```python
from build123d import *

# Parameters (mm, degrees)
F0_W           = 25.4
F0_H           = 76.2
F1_DEPTH       = 25.4
F2_W           = 25.4
F2_H           = 12.7
F3_DEPTH       = 6.35
F5_START       = -6.35
F4_R           = 9.525
F5_DEPTH       = 63.5
F6_R           = 5.1562
F7_DEPTH       = 76.201
F9_W           = 5.08
F9_H           = 76.2
F10_DEPTH      = 38.1
F11_W          = 20.32
F11_H          = 76.2
F12_DEPTH      = 6.35
F8_R           = 6.35
F13_DEPTH      = 5.6014842716
F13_DEPTH_BACK = 38.101


with BuildPart() as f1:
    # F0 (on Top) → F1 (new body)
    with BuildSketch(Plane.XY):
        with Locations((12.7, 38.1)):
            Rectangle(F0_W, F0_H)
    extrude(amount=F1_DEPTH)

    # F2 (on Top) → F3 (join)
    with BuildSketch(Plane.XY):
        with Locations((-12.7, 6.35)):
            Rectangle(F2_W, F2_H)
        with Locations((38.1, 6.35)):
            Rectangle(F2_W, F2_H)
        with Locations((-12.7, 69.85)):
            Rectangle(F2_W, F2_H)
        with Locations((38.1, 69.85)):
            Rectangle(F2_W, F2_H)
    extrude(amount=F3_DEPTH)

    # F4 (on face) → F5 (cut)
    with BuildSketch(Plane.XZ.offset(F5_START)):
        with Locations((12.7, 12.7)):
            Circle(F4_R)
    extrude(amount=-F5_DEPTH, mode=Mode.SUBTRACT)

    # F6 (on face) → F7 (cut, through all)
    with BuildSketch(Plane.XZ):
        with Locations((12.7, 12.7)):
            Circle(F6_R)
    extrude(amount=-F7_DEPTH, mode=Mode.SUBTRACT)

    # F9 (on face) → F10 (join)
    with BuildSketch(Plane.XY.offset(25.4)):
        with Locations((22.86, 38.1)):
            Rectangle(F9_W, F9_H)
        with Locations((2.54, 38.1)):
            Rectangle(F9_W, F9_H)
    extrude(amount=F10_DEPTH)

    # F11 (on face) → F12 (join)
    with BuildSketch(Plane.XY.offset(63.5)):
        with Locations((10.16, 38.1)):
            Rectangle(F11_W, F11_H)
    extrude(amount=-F12_DEPTH)

    # F8 (on face) → F13 (cut, two sides)
    with BuildSketch(Plane.XY.offset(25.4)) as f13_sk:
        with Locations((12.7, 38.1)):
            Circle(F8_R)
    extrude(amount=-F13_DEPTH, mode=Mode.SUBTRACT)
    extrude(f13_sk.sketch, amount=F13_DEPTH_BACK, mode=Mode.SUBTRACT)


solid = f1.part
```
Verification items for the finished model (mm, model axes). A direction names the side the tool comes from. Give positions to 0.01 mm unless a question says otherwise; leave off trailing zeros. Loops run counter-clockwise (first coordinate to the right, second up) from the corner with the lowest first, then second, coordinate; pieces in that order, holes last. Notation, with made-up numbers: M 19,56 L 36,56 A29 ccw 36,81 Z; hole C 34,88.25 d2. An arc over 180 degrees is marked long. One line per question, with ' | ' between items.
Item 1: Thickness scan on line 1 (X direction, y = 37.5, z = 30); line 2 (Z direction, x = 8.5, y = 59); line 3 (Z direction, x = 20, y = 46). Record the ranges inside material, lowest first. Write a range as [from, to].
Completed:
line 1: x = [0, 5.08], [20.32, 25.4] | line 2: z = [0, 4.15], [21.25, 25.4], [57.15, 63.5] | line 3: z = [0, 6.58], [18.82, 25.4], [57.15, 63.5]
Item 2: Section check B-B, the plane x = 33. Record the cut outline in (y, z).
Completed:
outline: M 0,0 L 12.7,0 L 12.7,6.35 L 0,6.35 Z; M 63.5,0 L 76.2,0 L 76.2,6.35 L 63.5,6.35 Z
Item 3: Section check A-A, the plane z = 12.7. Record the cut outline in (x, y) (3 decimals).
Completed:
outline: M 0,0 L 7.544,0 L 7.544,6.35 L 3.175,6.35 L 3.175,69.85 L 7.544,69.85 L 7.544,76.2 L 0,76.2 Z; M 17.856,0 L 25.4,0 L 25.4,76.2 L 17.856,76.2 L 17.856,69.85 L 22.225,69.85 L 22.225,6.35 L 17.856,6.35 Z
Item 4: Section check C-C, the plane y = 30. Record the cut outline in (x, z) (3 decimals).
Completed:
outline: M 0,0 L 25.4,0 L 25.4,63.5 L 0,63.5 Z; hole C 12.7,12.7 d19.05; hole M 5.08,25.4 L 20.32,25.4 L 20.32,57.15 L 5.08,57.15 Z
Item 5: Tool access check on faces 4 (the face through (19.4, 38.6, 57.15)), 5 (the face through (11.32, 31.9, 60.28)), 6 (the face through (38, 70, 6.35)), 7 (the face through (17, 6.35, 9)). Record the directions out of +Z, -Z, +X, -X, +Y, -Y that give a thin tool (end or side, any length) a straight path to the whole face; none if there is none.
Completed:
face 4: +Y, -Y | face 5: +Z | face 6: +Z, +X, +Y, -Y | face 7: none
Item 6: Draft check along Z on faces 1 (the face through (10.64, 37.66, 3.4)), 2 (the face through (10, 0, 25)), 3 (the face through (-13, 6, 6.35)). Enter one of: +Z half, -Z half, draft (parallel to the pull), parting line (faces both ways), or undercut.
Completed:
face 1: undercut | face 2: draft | face 3: +Z half
Item 7: Section check D-D, the plane x = 12.7. Record the cut outline in (y, z) (3 decimals), plus the area to 3 significant figures.
Completed:
outline: M 0,0 L 76.2,0 L 76.2,7.544 L 69.85,7.544 L 69.85,3.175 L 6.35,3.175 L 6.35,7.544 L 0,7.544 Z; M 0,17.856 L 6.35,17.856 L 6.35,22.225 L 31.75,22.225 L 31.75,25.4 L 0,25.4 Z; M 0,57.15 L 31.75,57.15 L 31.75,63.5 L 0,63.5 Z; M 44.45,22.225 L 69.85,22.225 L 69.85,17.856 L 76.2,17.856 L 76.2,25.4 L 44.45,25.4 Z; M 44.45,57.15 L 76.2,57.15 L 76.2,63.5 L 44.45,63.5 Z | area: 958 mm^2
Item 8: Depth check by flat-ended pin: P1, Ø6, axis at y = 35.5, z = 41.5, coming from the +X side; P2, Ø14, axis at x = 36, y = 9, coming from the +Z side. Enter the tip coordinate at first touch or a pass-through.
Completed:
P1: stops at x = 25.4 | P2: stops at z = 6.35
